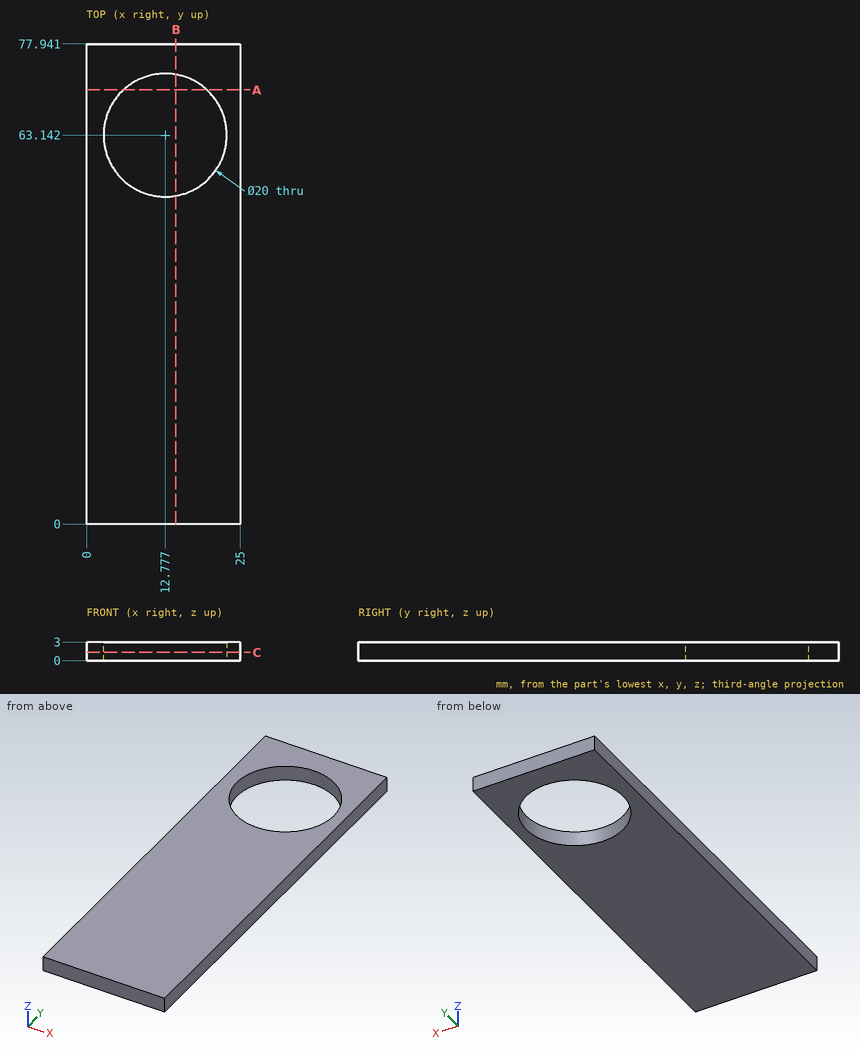
Source: three-view drawing plus pictorial views. Frame: mm from the lowest corner of the part. Give positions to 0.01 mm unless a question says otherwise; leave off trailing zeros. Order: outer loops, then holes, each group sorted by start corner. A loop starts at its lowest first (then second) coordinate and runs counter-clockwise, first axis right, second up. Notation, with made-up numbers: M 69,-14.75 L 89,-14.75 A21 ccw 89,20.25 Z; hole C 45.5,80 d7. An arc over 180 degrees is marked long. Return JSON: item names as keys, results as strings.
Item 1: Ray query, probe 1 along Y at (x, z) = (13, 0.45); probe 2 along Y at (x, z) = (19.5, 2.35) (1 decimal); probe 3 along X at (y, z) = (68.5, 0.7) (1 decimal). Return the intervals inside material, ascending.
Solutions:
{"probe 1": "0 to 53.14, 73.14 to 77.94", "probe 2": "0 to 55.7, 70.5 to 77.9", "probe 3": "0 to 4.3, 21.2 to 25"}
Item 2: Cut plane C-C (z = 1.3). Return loops of the section in (x, y).
Solutions:
{"outline": "M 0,0 L 25,0 L 25,77.94 L 0,77.94 Z; hole C 12.78,63.14 d20"}
Item 3: Cut plane B-B (x = 14.5). Return loops of the section in (y, z).
Solutions:
{"outline": "M 0,0 L 53.29,0 L 53.29,3 L 0,3 Z; M 72.99,0 L 77.94,0 L 77.94,3 L 72.99,3 Z"}
Item 4: Cut plane A-A (y = 70.5). Return loops of the section in (x, z) (1 decimal).
Solutions:
{"outline": "M 0,0 L 6,0 L 6,3 L 0,3 Z; M 19.5,0 L 25,0 L 25,3 L 19.5,3 Z"}
